Can you work these out from the model? Positions are in its coordinate system, mm. Face numbers are marked on the shaded views. A direction names the side the tool comes from. Round coordinates to 2 decimals unless told otherwise and drop trailing zeros. Write each loop counter-clockwise with the first axis right and the second up, starting at its lowest first coordinate (ties: lowest second). Pieces come first, ordered by that corner, then holes. Notation, with made-up numbers: M 52.5,9.5 L 103.5,9.5 A25 ccw 103.5,32.5 Z; hole C 70,-6.75 d1. An arc over 180 degrees is marked long. Use one line per item in the form item = value. Start each with the question number.
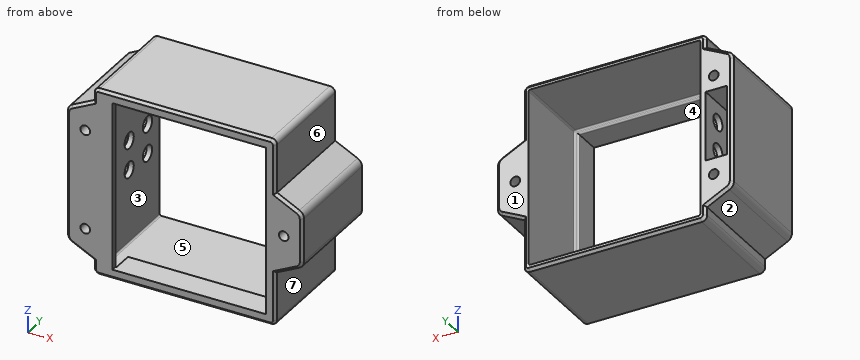
```python
from build123d import *

# Parameters (mm, degrees)
BOSS_EXTRUDE1_DEPTH = 40
SHELL1_START        = -33
SHELL1_OUTLINE_W    = 64
SHELL1_OUTLINE_H    = 38
SHELL1_DEPTH        = 66
SKETCH2_R           = 1.8
BOSS_EXTRUDE2_DEPTH = 40
CUT_EXTRUDE1_START  = 40
SKETCH3_W           = 8
SKETCH3_H           = 25.845374508
CUT_EXTRUDE1_DEPTH  = 38
SKETCH4_R           = 3
CUT_EXTRUDE2_DEPTH  = 2
SKETCH5_W           = 57.25
SKETCH5_H           = 62.7
CUT_EXTRUDE3_DEPTH  = 2
BOSS_EXTRUDE3_DEPTH = 8
CHAMFER1_SIZE       = 1
FILLET1_R           = 0.6


# Read off the part's stored shape, not the designer's step: Shell1
with BuildPart() as part:
    # Sketch1 → Boss-Extrude1 (new body)
    with BuildSketch(Plane(origin=(0, 0, 0), x_dir=(1, 0, 0), z_dir=(0, 1, 0))):
        with BuildLine():
            Line((-32, 35), (32, 35))
            ThreePointArc((32, 35), (33.414213562, 34.414213562), (34, 33))
            Line((34, 33), (34, -33))
            ThreePointArc((34, -33), (33.414213562, -34.414213562), (32, -35))
            Line((32, -35), (-32, -35))
            ThreePointArc((-32, -35), (-33.414213562, -34.414213562), (-34, -33))
            Line((-34, -33), (-34, 33))
            ThreePointArc((-34, 33), (-33.414213562, 34.414213562), (-32, 35))
        make_face()
    extrude(amount=BOSS_EXTRUDE1_DEPTH)

    # Shell1 outline → Shell1 (cut)
    with BuildSketch(Plane.XY.offset(SHELL1_START)):
        with Locations((0, 21)):
            Rectangle(SHELL1_OUTLINE_W, SHELL1_OUTLINE_H)
    extrude(amount=SHELL1_DEPTH, mode=Mode.SUBTRACT)

    # Sketch2 → Boss-Extrude2 (add)
    # profile 1 of 2: a face of its own
    with BuildSketch(Plane(origin=(0, 0, 0), x_dir=(1, 0, 0), z_dir=(0, 1, 0))):
        with BuildLine():
            Line((-34, 30), (-42.341640786, 25.829179607))
            ThreePointArc((-42.341640786, 25.829179607), (-43.551952425, 24.72309137), (-44, 23.145898034))
            Line((-44, 23.145898034), (-44, -23.145898034))
            ThreePointArc((-44, -23.145898034), (-43.551952425, -24.72309137), (-42.341640786, -25.829179607))
            Line((-42.341640786, -25.829179607), (-34, -30))
            Line((-34, -30), (-34, 30))
        make_face()
        with Locations(Location((-37, 18.896413475, 0), (0, 0, 90))):
            Circle(SKETCH2_R, mode=Mode.SUBTRACT)
        with Locations(Location((-37, -18.192906379, 0), (0, 0, 90))):
            Circle(SKETCH2_R, mode=Mode.SUBTRACT)
    # profile 2 of 2: a face of its own
    with BuildSketch(Plane(origin=(0, 0, 0), x_dir=(1, 0, 0), z_dir=(0, 1, 0))):
        with BuildLine():
            Line((34, 15), (42.341640786, 10.829179607))
            ThreePointArc((42.341640786, 10.829179607), (43.551952425, 9.72309137), (44, 8.145898034))
            Line((44, 8.145898034), (44, -8.145898034))
            ThreePointArc((44, -8.145898034), (43.551952425, -9.72309137), (42.341640786, -10.829179607))
            Line((42.341640786, -10.829179607), (34, -15))
            Line((34, -15), (34, 15))
        make_face()
        with Locations(Location((37, 0, 0), (0, 0, 90))):
            Circle(SKETCH2_R, mode=Mode.SUBTRACT)
    extrude(amount=BOSS_EXTRUDE2_DEPTH)

    # Sketch3 → Cut-Extrude1 (cut)
    with BuildSketch(Plane(origin=(0, 0, 0), x_dir=(1, 0, 0), z_dir=(0, 1, 0)).offset(CUT_EXTRUDE1_START)):
        with Locations((-38, 0)):
            Rectangle(SKETCH3_W, SKETCH3_H)
    extrude(amount=-CUT_EXTRUDE1_DEPTH, mode=Mode.SUBTRACT)

    # Sketch4 → Cut-Extrude2 (cut)
    with BuildSketch(Plane.ZY.offset(34)):
        with Locations((-5.5, 32)):
            Circle(SKETCH4_R)
        with Locations((5.5, 32)):
            Circle(SKETCH4_R)
        with Locations((-5.5, 20)):
            Circle(SKETCH4_R)
        with Locations((5.5, 20)):
            Circle(SKETCH4_R)
        with Locations((-5.5, 8)):
            Circle(SKETCH4_R)
        with Locations((5.5, 8)):
            Circle(SKETCH4_R)
    extrude(amount=-CUT_EXTRUDE2_DEPTH, mode=Mode.SUBTRACT)

    # Sketch5 → Cut-Extrude3 (cut)
    with BuildSketch(Plane(origin=(0, 0, 0), x_dir=(1, 0, 0), z_dir=(0, 1, 0))):
        with Locations((1.775, 0)):
            Rectangle(SKETCH5_W, SKETCH5_H)
    extrude(amount=CUT_EXTRUDE3_DEPTH, mode=Mode.SUBTRACT)

    # Sketch6 → Boss-Extrude3 (add)
    with BuildSketch(Plane(origin=(0, 2, 0), x_dir=(1, 0, 0), z_dir=(0, 1, 0))):
        Polygon((-26.85, 31.35), (-26.85, 33), (32, 33), (32, -33), (-26.85, -33), (-26.85, -31.35), (30.4, -31.35), (30.4, 31.35), align=None)
    extrude(amount=BOSS_EXTRUDE3_DEPTH)

    # Chamfer1
    chamfer1_edges = [part.edges().sort_by_distance(p)[0] for p in [
        (-34, 0, -31.5),
        (-33.414213562, 0, -34.414213562),
        (0, 0, -35),
        (33.414213562, 0, -34.414213562),
        (-33.414213562, 40, -34.414213562),
        (-34, 40, -31.5),
        (-33.414213562, 40, 34.414213562),
        (0, 40, 35),
        (33.414213562, 40, 34.414213562),
        (34, 40, 24),
        (-34, 0, 31.5),
        (-34, 40, 31.5),
        (-38.170820393, 40, -27.914589803),
        (-38.170820393, 0, -27.914589803),
        (-43.551952425, 40, -24.72309137),
        (-43.551952425, 0, -24.72309137),
        (-44, 40, 0),
        (-44, 0, 0),
        (-43.551952425, 40, 24.72309137),
        (-43.551952425, 0, 24.72309137),
        (-38.170820393, 40, 27.914589803),
        (-38.170820393, 0, 27.914589803),
        (33.414213562, 40, -34.414213562),
        (34, 0, -24),
        (34, 40, -24),
        (38.170820393, 40, 12.914589803),
        (38.170820393, 0, 12.914589803),
        (43.551952425, 40, 9.72309137),
        (43.551952425, 0, 9.72309137),
        (44, 40, 0),
        (44, 0, 0),
        (43.551952425, 40, -9.72309137),
        (43.551952425, 0, -9.72309137),
        (38.170820393, 40, -12.914589803),
        (38.170820393, 0, -12.914589803),
        (34, 0, 24),
        (0, 40, -35),
        (33.414213562, 0, 34.414213562),
        (0, 0, 35),
        (-33.414213562, 0, 34.414213562),
    ]]
    chamfer(chamfer1_edges, length=CHAMFER1_SIZE)

    # Fillet1
    fillet1_edges = [part.edges().sort_by_distance(p)[0] for p in [
        (-29.425, 2, -33),
        (-26.85, 6, -31.35),
        (-26.85, 6, 31.35),
        (-26.85, 6, 33),
        (-26.85, 6, -33),
        (1.775, 10, -31.35),
        (30.4, 10, 0),
        (1.775, 10, 31.35),
        (2.575, 10, 33),
        (32, 10, 0),
        (2.575, 10, -33),
        (32, 25, -33),
        (-32, 2, 0),
        (-32, 21, -33),
        (-29.425, 2, 33),
        (-32, 21, 33),
        (32, 25, 33),
    ]]
    fillet(fillet1_edges, radius=FILLET1_R)


solid = part.part
```
1. Please list where these lines run through material, in increasing order: line 1 along X through (y, z) = (32, -19); line 2 along Y through (x, z) = (-33.25, 5.5); line 3 along X through (y, z) = (14, 23).
2. Will these pins go through, and if not, where does the flat tip stop? pin 1 (4 mm diameter, centred on x = -28.5, z = -2, fed in from +Y); pin 2 (9 mm diameter, centred on x = -39, y = 13.5, fed in from +Z).
3. If we section it at A-A (z = 0): List the corners of the cut face in (x, y) for me, and give its area (3 significant figures).
4. If we section it at B-B (y = 20): State how many separate pieces and enclosed holes the cut face has, and give its area (3 significant figures).
5. If we section it at D-D (z = -27): List the corners of the cut face in (x, y) for me, and give its area (3 significant figures).
6. If we mould it in two halves opening along X, with no side actions, what happens to the marked faces 1, 2 and 3? For each: pulls with the +X half, pulls with the -X half, needs draft (parallel to the pull), parting line crosses it, or undercut.
7. Which directions (+Z, -Z, +X, -X, +Y, -Y) give clear straight access to the entire face, cutting with the end or side of a thin tool? Please do the marked faces 4, 5, 6 and 7.
8. If we section it at C-C (x = 26): List the corners of the cut face in (y, z) for me.
Model answer:
q1.line_1 = -44 to -38.8, -35.2 to -32, 32 to 34
q1.line_2 = 0 to 5, 11 to 17, 23 to 29, 35 to 40
q1.line_3 = -44 to -32, 32 to 34
q2.pin_1 = 2
q2.pin_2 = 29.75
q3.outline = M -44,1 L -43,0 L -26.85,0 L -26.85,2 L -31.4,2 A0.6 cw -32,2.6 L -32,40 L -34,40 L -34,2 L -42,2 L -42,40 L -43,40 L -44,39 Z; M 30.4,0 L 35.2,0 L 35.2,40 L 32,40 L 32,10.6 A0.6 cw 31.4,10 L 31,10 A0.6 ccw 30.4,9.4 Z; M 38.8,0 L 43,0 L 44,1 L 44,39 L 43,40 L 38.8,40 Z
q3.area = 536 mm2
q4.separate_pieces = 2
q4.enclosed_holes = 4
q4.area = 1,070 mm2
q5.outline = M -40,1 L -37.76,0 L -26.85,0 L -26.85,2 L -31.4,2 A0.6 cw -32,2.6 L -32,40 L -37.76,40 L -40,39 Z; M 30.4,0 L 33,0 L 34,1 L 34,39 L 33,40 L 32,40 L 32,10.6 A0.6 cw 31.4,10 L 31,10 A0.6 ccw 30.4,9.4 Z
q5.area = 423 mm2
q6.face_1 = needs draft
q6.face_2 = pulls with the -X half
q6.face_3 = undercut
q7.face_4 = +Y, -Y
q7.face_5 = +Y
q7.face_6 = +Z, +X, +Y, -Y
q7.face_7 = -Z, +X, +Y, -Y
q8.outline = M 0,-34 L 1,-35 L 39,-35 L 40,-34 L 40,-33 L 10.6,-33 A0.6 cw 10,-32.4 L 10,-31.95 A0.6 ccw 9.4,-31.35 L 0,-31.35 Z; M 0,31.35 L 9.4,31.35 A0.6 ccw 10,31.95 L 10,32.4 A0.6 cw 10.6,33 L 40,33 L 40,34 L 39,35 L 1,35 L 0,34 Z
